Design review of the part built by this model. Coordinates are the model's own, in mm. Coordinates: 2 decimals unless noted, no trailing zeros. Write each loop counter-clockwise with the first axis right and the second up, starting at its lowest first coordinate (ties: lowest second). Pieces come first, ordered by that corner, then holes. Notation, with made-up numbers: (42, 75) - (76, 75) arc R12 cw to (76, 97) - close; hole circle Ø2 at (24.5, 25). An arc over 180 degrees is marked (long way). Use a Markdown table: item, result.
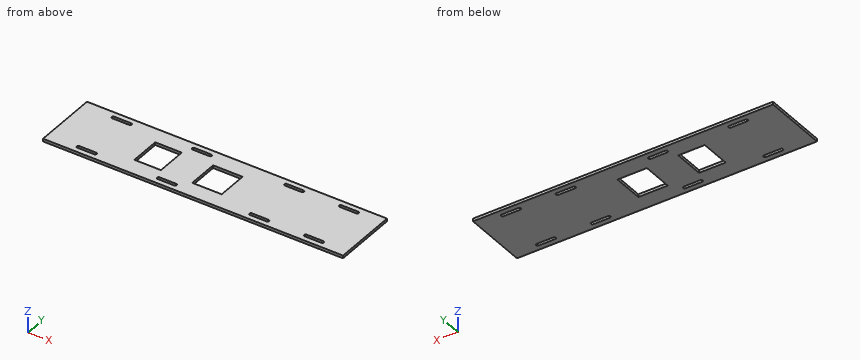
from build123d import *

# Parameters (mm, degrees)
F0_W     = 25.5
F0_H     = 26.5
F0_W_2   = 23
F1_DEPTH = 2.4


with BuildPart() as f1:
    # F0 (on Top) → F1 (new body)
    with BuildSketch(Plane.XY):
        Polygon((109.5, -28), (130, -28), (130, 28), (109.5, 28), (-35, 28), (-61, 28), (-104.5, 28), (-130, 28), (-130, -28), (-104.5, -28), (-35, -28), (-10.5, -28), (62, -28), align=None)
        with BuildLine():
            Line((-88.75, -23.5), (-103.25, -23.5))
            ThreePointArc((-103.25, -23.5), (-104.133883, -23.133883), (-104.5, -22.25))
            ThreePointArc((-104.5, -22.25), (-104.133883, -21.366117), (-103.25, -21))
            Line((-103.25, -21), (-88.75, -21))
            ThreePointArc((-88.75, -21), (-87.866117, -21.366117), (-87.5, -22.25))
            ThreePointArc((-87.5, -22.25), (-87.866117, -23.133883), (-88.75, -23.5))
        make_face(mode=Mode.SUBTRACT)
        with BuildLine():
            Line((-19.25, -23.5), (-33.75, -23.5))
            ThreePointArc((-33.75, -23.5), (-34.633883, -23.133883), (-35, -22.25))
            ThreePointArc((-35, -22.25), (-34.633883, -21.366117), (-33.75, -21))
            Line((-33.75, -21), (-19.25, -21))
            ThreePointArc((-19.25, -21), (-18.366117, -21.366117), (-18, -22.25))
            ThreePointArc((-18, -22.25), (-18.366117, -23.133883), (-19.25, -23.5))
        make_face(mode=Mode.SUBTRACT)
        with BuildLine():
            ThreePointArc((62, -22.25), (61.633883, -23.133883), (60.75, -23.5))
            Line((60.75, -23.5), (46.25, -23.5))
            ThreePointArc((46.25, -23.5), (45.366117, -23.133883), (45, -22.25))
            ThreePointArc((45, -22.25), (45.366117, -21.366117), (46.25, -21))
            Line((46.25, -21), (60.75, -21))
            ThreePointArc((60.75, -21), (61.633883, -21.366117), (62, -22.25))
        make_face(mode=Mode.SUBTRACT)
        with BuildLine():
            ThreePointArc((109.5, -22.25), (109.133883, -23.133883), (108.25, -23.5))
            Line((108.25, -23.5), (93.75, -23.5))
            ThreePointArc((93.75, -23.5), (92.866117, -23.133883), (92.5, -22.25))
            ThreePointArc((92.5, -22.25), (92.866117, -21.366117), (93.75, -21))
            Line((93.75, -21), (108.25, -21))
            ThreePointArc((108.25, -21), (109.133883, -21.366117), (109.5, -22.25))
        make_face(mode=Mode.SUBTRACT)
        with Locations((2.25, -0.25)):
            Rectangle(F0_W, F0_H, mode=Mode.SUBTRACT)
        with Locations((-49.5, 0.25)):
            Rectangle(F0_W_2, F0_H, mode=Mode.SUBTRACT)
        with BuildLine():
            ThreePointArc((-104.5, 22.25), (-104.133883, 23.133883), (-103.25, 23.5))
            Line((-103.25, 23.5), (-88.5, 23.5))
            ThreePointArc((-88.5, 23.5), (-87.792893, 23.207107), (-87.5, 22.5))
            Line((-87.5, 22.5), (-87.5, 22.25))
            ThreePointArc((-87.5, 22.25), (-87.866117, 21.366117), (-88.75, 21))
            Line((-88.75, 21), (-103.25, 21))
            ThreePointArc((-103.25, 21), (-104.133883, 21.366117), (-104.5, 22.25))
        make_face(mode=Mode.SUBTRACT)
        with BuildLine():
            ThreePointArc((-35, 22.25), (-34.633883, 23.133883), (-33.75, 23.5))
            Line((-33.75, 23.5), (-19.25, 23.5))
            ThreePointArc((-19.25, 23.5), (-18.366117, 23.133883), (-18, 22.25))
            ThreePointArc((-18, 22.25), (-18.366117, 21.366117), (-19.25, 21))
            Line((-19.25, 21), (-33.75, 21))
            ThreePointArc((-33.75, 21), (-34.633883, 21.366117), (-35, 22.25))
        make_face(mode=Mode.SUBTRACT)
        with BuildLine():
            Line((46.25, 23.5), (60.75, 23.5))
            ThreePointArc((60.75, 23.5), (61.633883, 23.133883), (62, 22.25))
            ThreePointArc((62, 22.25), (61.633883, 21.366117), (60.75, 21))
            Line((60.75, 21), (46.25, 21))
            ThreePointArc((46.25, 21), (45.366117, 21.366117), (45, 22.25))
            ThreePointArc((45, 22.25), (45.366117, 23.133883), (46.25, 23.5))
        make_face(mode=Mode.SUBTRACT)
        with BuildLine():
            Line((93.75, 23.5), (108.25, 23.5))
            ThreePointArc((108.25, 23.5), (109.133883, 23.133883), (109.5, 22.25))
            ThreePointArc((109.5, 22.25), (109.133883, 21.366117), (108.25, 21))
            Line((108.25, 21), (93.75, 21))
            ThreePointArc((93.75, 21), (92.866117, 21.366117), (92.5, 22.25))
            ThreePointArc((92.5, 22.25), (92.866117, 23.133883), (93.75, 23.5))
        make_face(mode=Mode.SUBTRACT)
    extrude(amount=F1_DEPTH)


solid = f1.part
(1) For L1, parallel to Y at x = 96, z = 1.05; L2, parallel to X at y = -1.5, z = 2.2; L3, parallel to Y at x = 8, z = 0.25, list the stretches that pass through material, from the lowest coordinate up. Write a range as from..to.
Determined:
| item | result |
|---|---|
| L1 | -28..-23.5, -21..21, 23.5..28 |
| L2 | -130..-61, -38..-10.5, 15..130 |
| L3 | -28..-13.5, 13..28 |
(2) Take a section at C-C on x = -46. Write out the cut boundary in (y, z), and give its area (3 significant figures).
Determined:
| item | result |
|---|---|
| outline | (-28, 0) - (-13, 0) - (-13, 2.4) - (-28, 2.4) - close; (13.5, 0) - (28, 0) - (28, 2.4) - (13.5, 2.4) - close |
| area | 70.8 mm2 |
(3) Take a section at A-A on x = 97. Write out the cut boundary in (y, z), and give its area (3 significant figures).
Determined:
| item | result |
|---|---|
| outline | (-28, 0) - (-23.5, 0) - (-23.5, 2.4) - (-28, 2.4) - close; (-21, 0) - (21, 0) - (21, 2.4) - (-21, 2.4) - close; (23.5, 0) - (28, 0) - (28, 2.4) - (23.5, 2.4) - close |
| area | 122 mm2 |
(4) Take a section at D-D on z = 1.4. State how many separate pieces and enclosed holes the cut face has, and give its area (3 significant figures).
Determined:
| item | result |
|---|---|
| separate pieces | 1 |
| enclosed holes | 10 |
| area | 12,900 mm2 |
(5) Take a section at B-B on y = 10.5. Write out the cut boundary in (x, z).
Determined:
| item | result |
|---|---|
| outline | (-130, 0) - (-61, 0) - (-61, 2.4) - (-130, 2.4) - close; (-38, 0) - (-10.5, 0) - (-10.5, 2.4) - (-38, 2.4) - close; (15, 0) - (130, 0) - (130, 2.4) - (15, 2.4) - close |
